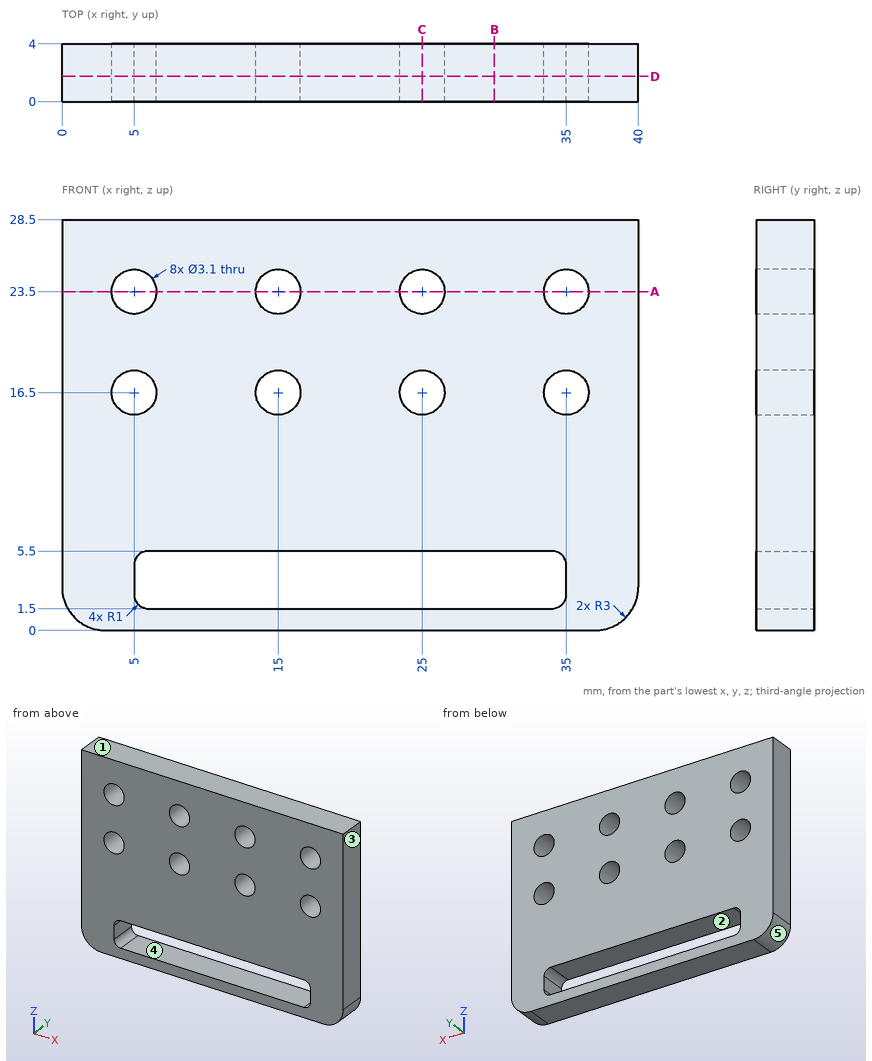
The drawing under review shows one solid part. Ordinate dimensions are in mm from its lowest x, y, z. A direction names the side the tool comes from. Give positions to 0.01 mm unless a question says otherwise; leave off trailing zeros. Loops run counter-clockwise (first coordinate to the right, second up) from the corner with the lowest first, then second, coordinate; pieces in that order, holes last. Notation, with made-up numbers: M 88,-25.5 L 111,-25.5 A4 ccw 111,-21.5 Z; hole C 17,62.5 d4. An arc over 180 degrees is marked long. One line per item, written item: value. Start each with the question number.
Q1. Add section D-D (y = 1.75). Count the separate pieces of the cut face and the enclosed holes in it, and give its area (3 significant figures).
Q2. For L1, parallel to X at y = 2.65, z = 23.5; L2, parallel to Z at x = 32, y = 1.55; L3, parallel to Z at x = 6, y = 0.65, list the stretches that pass through material, from the lowest coordinate up.
Q3. Clearance check with a flat-ended pin moving along its axis: pin 1 Ø2.5 at (x, z) = (5, 23.5) entering from +Y. State where the tip first meets the part, or that it passes through.
Q4. Add section A-A (z = 23.5). Give the boundary of the cut face in (x, y), and give its area (3 significant figures).
Q5. Machinability: for the marked faces 4 and 5, which of the approach directions +Z, -Z, +X, -X, +Y, -Y give a long, thin tool a straight path to every point of the face, cutting with its end or side? Answer none if there is none.
Q6. Add section B-B (x = 30). Give the boundary of the cut face in (y, z), and give its area (3 significant figures).
Q7. Add section C-C (x = 25). Give the boundary of the cut face in (y, z).
Q8. Draft analysis for pull direction X (two halves, no side actions). For the marked faces 1, 2 and 3, state which applies: released by +X, released by -X, zero draft, split by the parting line, or undercut.
Reply:
1. separate pieces: 1
1. enclosed holes: 9
1. area: 957 mm²
2. L1: 0 to 3.45, 6.55 to 13.45, 16.55 to 23.45, 26.55 to 33.45, 36.55 to 40
2. L2: 0 to 1.5, 5.5 to 28.5
2. L3: 0 to 1.5, 5.5 to 15.32, 17.68 to 22.32, 24.68 to 28.5
3. pin 1: through
4. outline: M 0,0 L 3.45,0 L 3.45,4 L 0,4 Z; M 6.55,0 L 13.45,0 L 13.45,4 L 6.55,4 Z; M 16.55,0 L 23.45,0 L 23.45,4 L 16.55,4 Z; M 26.55,0 L 33.45,0 L 33.45,4 L 26.55,4 Z; M 36.55,0 L 40,0 L 40,4 L 36.55,4 Z
4. area: 110 mm²
5. face 4: +Y, -Y
5. face 5: -Z, -X, +Y, -Y
6. outline: M 0,0 L 4,0 L 4,1.5 L 0,1.5 Z; M 0,5.5 L 4,5.5 L 4,28.5 L 0,28.5 Z
6. area: 98.0 mm²
7. outline: M 0,0 L 4,0 L 4,1.5 L 0,1.5 Z; M 0,5.5 L 4,5.5 L 4,14.95 L 0,14.95 Z; M 0,18.05 L 4,18.05 L 4,21.95 L 0,21.95 Z; M 0,25.05 L 4,25.05 L 4,28.5 L 0,28.5 Z
8. face 1: zero draft
8. face 2: undercut
8. face 3: released by +X
